Verification items for the finished model (mm, model axes). Face numbers are marked on the shaded views. Round coordinates to 2 decimals unless told otherwise and drop trailing zeros. Order: outer loops, then holes, each group sorted by start corner. A loop starts at its lowest first (then second) coordinate and runs counter-clockwise, first axis right, second up. Notation, with made-up numbers: (-0.5, 48) -> (38.5, 48) arc R6 ccw to (38.5, 54) -> close; hole circle Ø5 at (78.25, -14). An arc over 180 degrees is marked (long way). Put each result on its own line as item: value.
```python
from build123d import *

# Parameters (mm, degrees)
R_P_TITION_CIRCULAIRE1_COUNT = 4
ENL_V_MAT_EXTRU_1_DEPTH      = 2.1
ENL_V_MAT_EXTRU_2_DEPTH      = 2


with BuildPart() as part:
    # Esquisse1 → Révolution1 (revolve)
    with BuildSketch(Plane.XY):
        with BuildLine():
            Line((0, 2.8), (0, 23.375))
            ThreePointArc((0, 23.375), (0.146446609, 23.728553391), (0.5, 23.875))
            Line((0.5, 23.875), (5.5, 23.875))
            Line((5.5, 23.875), (5.5, 23.375))
            Line((5.5, 23.375), (6, 23.375))
            Line((6, 23.375), (6, 23.875))
            Line((6, 23.875), (14, 23.875))
            Line((14, 23.875), (14, 23.375))
            Line((14, 23.375), (14.5, 23.375))
            Line((14.5, 23.375), (14.5, 23.875))
            Line((14.5, 23.875), (19.5, 23.875))
            ThreePointArc((19.5, 23.875), (19.853553391, 23.728553391), (20, 23.375))
            Line((20, 23.375), (20, 7.1))
            Line((20, 7.1), (17, 7.1))
            Line((17, 7.1), (17, 4))
            Line((17, 4), (20, 4))
            Line((20, 4), (20, 2.8))
            Line((20, 2.8), (0, 2.8))
        make_face()
    revolve(axis=Axis((-88.596801802, 0, 0), (1, 0, 0)))

    # Esquisse4 → Dégagement M2.51 (revolve, cut)
    with BuildSketch(Plane.ZX.offset(7.5)):
        Polygon((0, 0), (0, 3.371247898), (1.45, 2.5), (1.45, 0), align=None)
    d_gagement_m2_51 = revolve(axis=Axis((-6.35, 7.5, 0), (1, 0, 0)), mode=Mode.SUBTRACT)

    # Esquisse7 → Dégagement M31 (revolve, cut)
    with BuildSketch(Plane(origin=(20, 8.838834765, 8.838834765), x_dir=(0, 0, -1), z_dir=(0, 1, 0))):
        Polygon((0, 0), (0, 3.521463052), (1.7, 2.5), (1.7, 0), align=None)
    d_gagement_m31 = revolve(axis=Axis((26.35, 8.838834765, 8.838834765), (-1, 0, 0)), mode=Mode.SUBTRACT)

    # Répétition circulaire1: Dégagement M2.51, Dégagement M31 ×4 about axis
    r_p_tition_circulaire1_axis = Axis((0, 0, 0), (1, 0, 0))
    for i in range(1, R_P_TITION_CIRCULAIRE1_COUNT):
        add(d_gagement_m2_51.rotate(r_p_tition_circulaire1_axis, i * 360 / R_P_TITION_CIRCULAIRE1_COUNT), mode=Mode.SUBTRACT)
        add(d_gagement_m31.rotate(r_p_tition_circulaire1_axis, i * 360 / R_P_TITION_CIRCULAIRE1_COUNT), mode=Mode.SUBTRACT)

    # Esquisse9 → Enlèv. mat.-Extru.1 (cut)
    with BuildSketch(Plane(origin=(20, 0, 0), x_dir=(0, 0, -1), z_dir=(1, 0, 0))):
        with BuildLine():
            Line((2.75, 13.282856857), (2.25, 13.282856857))
            ThreePointArc((2.25, 13.282856857), (1.896446609, 13.429303466), (1.75, 13.782856857))
            Line((1.75, 13.782856857), (1.75, 14.782856857))
            ThreePointArc((1.75, 14.782856857), (1.896446609, 15.136410248), (2.25, 15.282856857))
            Line((2.25, 15.282856857), (2.75, 15.282856857))
            ThreePointArc((2.75, 15.282856857), (3.103553391, 15.136410248), (3.25, 14.782856857))
            Line((3.25, 14.782856857), (3.25, 13.782856857))
            ThreePointArc((3.25, 13.782856857), (3.103553391, 13.429303466), (2.75, 13.282856857))
        make_face()
        with BuildLine():
            Line((0.25, 13.282856857), (-0.25, 13.282856857))
            ThreePointArc((-0.25, 13.282856857), (-0.603553391, 13.429303466), (-0.75, 13.782856857))
            Line((-0.75, 13.782856857), (-0.75, 14.782856857))
            ThreePointArc((-0.75, 14.782856857), (-0.603553391, 15.136410248), (-0.25, 15.282856857))
            Line((-0.25, 15.282856857), (0.25, 15.282856857))
            ThreePointArc((0.25, 15.282856857), (0.603553391, 15.136410248), (0.75, 14.782856857))
            Line((0.75, 14.782856857), (0.75, 13.782856857))
            ThreePointArc((0.75, 13.782856857), (0.603553391, 13.429303466), (0.25, 13.282856857))
        make_face()
        with BuildLine():
            Line((-2.25, 13.282856857), (-2.75, 13.282856857))
            ThreePointArc((-2.75, 13.282856857), (-3.103553391, 13.429303466), (-3.25, 13.782856857))
            Line((-3.25, 13.782856857), (-3.25, 14.782856857))
            ThreePointArc((-3.25, 14.782856857), (-3.103553391, 15.136410248), (-2.75, 15.282856857))
            Line((-2.75, 15.282856857), (-2.25, 15.282856857))
            ThreePointArc((-2.25, 15.282856857), (-1.896446609, 15.136410248), (-1.75, 14.782856857))
            Line((-1.75, 14.782856857), (-1.75, 13.782856857))
            ThreePointArc((-1.75, 13.782856857), (-1.896446609, 13.429303466), (-2.25, 13.282856857))
        make_face()
    extrude(amount=-ENL_V_MAT_EXTRU_1_DEPTH, mode=Mode.SUBTRACT)

    # Esquisse10 → Enlèv. mat.-Extru.2 (cut)
    with BuildSketch(Plane(origin=(20, 0, 0), x_dir=(0, 0, -1), z_dir=(1, 0, 0))):
        with BuildLine():
            Line((3.75, 22.642948682), (3.75, 13.782856857))
            ThreePointArc((3.75, 13.782856857), (3.457106781, 13.075750076), (2.75, 12.782856857))
            Line((2.75, 12.782856857), (-2.75, 12.782856857))
            ThreePointArc((-2.75, 12.782856857), (-3.457106781, 13.075750076), (-3.75, 13.782856857))
            Line((-3.75, 13.782856857), (-3.75, 22.642948682))
            ThreePointArc((-3.75, 22.642948682), (-3.627835365, 22.970424539), (-3.321038251, 23.137876522))
            ThreePointArc((-3.321038251, 23.137876522), (0, 23.375), (3.321038251, 23.137876522))
            ThreePointArc((3.321038251, 23.137876522), (3.627835365, 22.970424539), (3.75, 22.642948682))
        make_face()
    extrude(amount=-ENL_V_MAT_EXTRU_2_DEPTH, mode=Mode.SUBTRACT)


solid = part.part
```
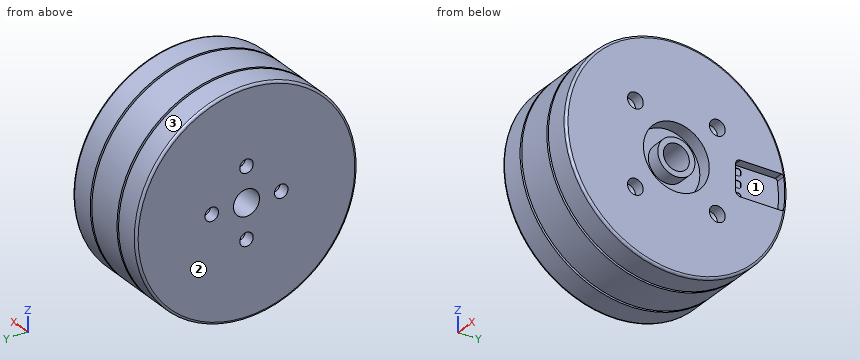
Item 1: Sectioned sample at A-A, the plane x = 13.25. Record the boundary of the cut face in (y, z) (3 decimals).
Geometry check:
outline: circle Ø47.75 at (0, 0); hole circle Ø5.6 at (0, 0)
Item 2: Release check for a two-part mould opening along Z. For the marked faces 1, 2 and 3 record: pulls with the +Z half, pulls with the -Z half, needs draft (parallel to the pull), parting line crosses it, or undercut.
Geometry check:
face 1: undercut
face 2: needs draft
face 3: parting line crosses it
Item 3: Depth check by flat-ended pin: pin 1 Ø3 at (x, z) = (7.5, -13) entering from -Y; pin 2 Ø1.6 at (y, z) = (14, 0) entering from +X; pin 3 Ø1.5 at (x, z) = (14, -18.5) entering from -Y; pin 4 Ø24 at (y, z) = (-5.5, 4) entering from -X. Enter the tip coordinate at first touch or a pass-through.
Geometry check:
pin 1: y = -20.92
pin 2: x = 18
pin 3: y = -15.97
pin 4: x = 0
Item 4: Material ranges on line 1 along Z through (x, y) = (1.4, 0) (3 decimals); line 2 along Z through (x, y) = (17.75, -2.5); line 3 along Y through (x, z) = (2.25, 7), recorded low to high.
Geometry check:
line 1: -23.875 to -8.95, -6.05 to -2.8, 2.8 to 6.05, 8.95 to 23.875
line 2: -23.74 to -6.65, -3.12 to -1.26, 1.26 to 3.12, 6.65 to 23.74
line 3: -22.83 to -1.36, 1.36 to 22.83
